Autodesk Inventor part; units mm, degrees
ref_plane "YZ Plane" through (0, 0, 0) normal (1, 0, 0) x (0, 1, 0)
ref_plane "XZ Plane" through (0, 0, 0) normal (0, 1, 0) x (-1, 0, 0)
ref_plane "XY Plane" through (0, 0, 0) normal (0, 0, 1) x (1, 0, 0)
sketch "Sketch1" plane through (0, 0, 0) normal (0, 0, 1) x (1, 0, 0)
  circle A0 centre (-4064, 0) radius 361.95
  circle A1 centre (-4064, 0) radius 412.75
  line L0 (0, -577.85) -> (0, 577.85)
  point P0 (0, 0)
  dimension "d0" = 723.9
  dimension "d1" = 825.5
  dimension "d2" = 4064
revolve "Revolution1" add sketch "Sketch1" angle 30 about axis through (0, -10, 0) along (0, 1, 0)
sketch "Sketch10" plane through (-4064, 0, 0) normal (0, 0, -1) x (-1, 0, 0)
  circle A0 centre (0, 0) radius 387.35
  circle A1 centre (0, 0) radius 412.75 construction
  point P0 (-4064, 0)
  dimension "d34" = 774.7
extrude "Extrusion9" cut sketch "Sketch10" against normal blind 12.7
sketch "Sketch11" plane through (-3519.5272, 0, 2032) normal (0.5, 0, 0.8660254) x (0.8660254, 0, -0.5)
  circle A0 centre (0, 0) radius 387.35
  line L0 (4064, -577.85) -> (4064, 577.85)
  circle A1 centre (0, 0) radius 412.75
  point P0 (4064, 0)
  dimension "d37" = 774.7
revolve "Revolution3" add sketch "Sketch11" angle 0.5 about axis through (0, -10, 0) along (0, 1, 0) contours A0 | A1
extrude "Extrusion10" cut sketch "Sketch11" against normal blind 6.35 contours A0
extrude "Extrusion12" cut sketch "Sketch11" along normal blind 6.35 contours A0
sketch "Sketch12" plane through (-3516.3522, 0, 2037.4993) normal (-0.5, 0, -0.8660254) x (-0.8660254, 0, 0.5)
  circle A0 centre (0, 0) radius 387.35 construction
  circle A1 centre (0, 0) radius 463.55
  point P0 (-4064, 0)
  dimension "d52" = 927.1
extrude "Extrusion13" cut sketch "Sketch12" against normal through all
fillet "Fillet3" radius 0.7937 2 edges at (-3858.1582, 0, 2220.174) (-3676.65, 0, 12.7)
chamfer "Chamfer3" distance 0.7937 angle 45 2 edges at (-3851.8072, 0, 2231.1743) (-3676.65, 0, 0)
properties part number "A1-19027-100-05 HCWI elbow - female" material "Iron, HCWI"
Model file for the job. Use its own axes, mm. A direction names the side the tool comes from. Give positions to 0.01 mm unless a question says otherwise; leave off trailing zeros.
1) Mould opens along Y. For faces 1 (the cylindrical face through (-3199.52, 116.35, 1847.34)), 2 (the flat face through (-3760, -243, 0)) say: +Y half, -Y half, draft (parallel to the pull), parting line (faces both ways), or undercut.
2) 3-axis set-ups, long thin cutter, end or side, ignore diameter. For faces 3 (the flat face through (-3753.07, 277.33, 2174.17)), 4 (the cylindrical face through (-3677.025, 17.031, 6.272)): which of +Z, -Z, +X, -X, +Y, -Y reach the whole face in a straight line?
3) Wall check: probe 1 along Y at (x, z) = (-4064, 4.5); probe 2 along Y at (x, z) = (-3604.5, 1045); probe 3 along X at (y, z) = (73.5, 253). Give the ranges that are in metal, low to high.
4) Pin check, flat tips, straight feed: pin 1 (3 mm diameter, centred on x = -3949.5, z = 1395, fed in from -Y); pin 2 (4 mm diameter, centred on y = -77.5, z = 726, fed in from -X); pin 3 (3 mm diameter, centred on y = -71.5, z = 968.5, fed in from +X). Stop position of each tip, or through.
Computed:
1. face 1: undercut
1. face 2: draft
2. face 3: +Z, +X, +Y, -Y
2. face 4: -Z
3. probe 1: y = -412.75 to -387.35, 387.35 to 412.75
3. probe 2: y = -271.28 to -185.04, 185.04 to 271.28
3. probe 3: x = -4462.99 to -4411.16, -3700.95 to -3649.09
4. pin 1: stops at y = -393.96
4. pin 2: stops at x = -4410.56
4. pin 3: stops at x = -3526.44
